```python
from build123d import *

# Parameters (mm, degrees)
BASE_FLANGE1_DEPTH = 490.75
CUT_EXTRUDE2_DEPTH = 514.204272196


# Sheet-metal steps are written as plain solids
with BuildPart() as part:
    # Sketch1 → Base-Flange1 (new, symmetric)
    with BuildSketch(Plane(origin=(0, 0, 0), x_dir=(1, 0, 0), z_dir=(0, 1, 0))):
        with BuildLine():
            Line((9.5, 58), (9.5, 68.0134))
            ThreePointArc((9.5, 68.0134), (10.081861668, 69.418138332), (11.4866, 70))
            Line((11.4866, 70), (37.5134, 70))
            ThreePointArc((37.5134, 70), (38.918138332, 69.418138332), (39.5, 68.0134))
            Line((39.5, 68.0134), (39.5, 23))
            Line((39.5, 23), (39.5, 18))
            Line((39.5, 18), (39.5, 7.8))
            ThreePointArc((39.5, 7.8), (41.269678139, 6.091041686), (42.915834526, 7.91928357))
            Line((42.915834526, 7.91928357), (42.359529101, 15.874821789))
            ThreePointArc((42.359529101, 15.874821789), (42.88838258, 17.368257942), (44.341289843, 18))
            Line((44.341289843, 18), (52.2634, 18))
            ThreePointArc((52.2634, 18), (53.668138332, 17.418138332), (54.25, 16.0134))
            Line((54.25, 16.0134), (54.25, -21.0134))
            ThreePointArc((54.25, -21.0134), (53.668138332, -22.418138332), (52.2634, -23))
            Line((52.2634, -23), (40.2366, -23))
            ThreePointArc((40.2366, -23), (39.715745145, -23.215745145), (39.5, -23.7366))
            Line((39.5, -23.7366), (39.5, -68.0134))
            ThreePointArc((39.5, -68.0134), (38.918138332, -69.418138332), (37.5134, -70))
            Line((37.5134, -70), (11.4866, -70))
            ThreePointArc((11.4866, -70), (10.081861668, -69.418138332), (9.5, -68.0134))
            Line((9.5, -68.0134), (9.5, -58))
            Line((9.5, -58), (10.75, -58))
            Line((10.75, -58), (10.75, -68.0134))
            ThreePointArc((10.75, -68.0134), (10.965745145, -68.534254855), (11.4866, -68.75))
            Line((11.4866, -68.75), (37.5134, -68.75))
            ThreePointArc((37.5134, -68.75), (38.034254855, -68.534254855), (38.25, -68.0134))
            Line((38.25, -68.0134), (38.25, -23.7366))
            ThreePointArc((38.25, -23.7366), (38.831861668, -22.331861668), (40.2366, -21.75))
            Line((40.2366, -21.75), (52.2634, -21.75))
            ThreePointArc((52.2634, -21.75), (52.784254855, -21.534254855), (53, -21.0134))
            Line((53, -21.0134), (53, 16.0134))
            ThreePointArc((53, 16.0134), (52.784254855, 16.534254855), (52.2634, 16.75))
            Line((52.2634, 16.75), (44.341289843, 16.75))
            ThreePointArc((44.341289843, 16.75), (43.802574707, 16.515759992), (43.606484164, 15.962017381))
            Line((43.606484164, 15.962017381), (44.162789589, 8.006479162))
            ThreePointArc((44.162789589, 8.006479162), (41.31330251, 4.841803152), (38.25, 7.8))
            Line((38.25, 7.8), (38.25, 18))
            Line((38.25, 18), (38.25, 23))
            Line((38.25, 23), (38.25, 68.0134))
            ThreePointArc((38.25, 68.0134), (38.034254855, 68.534254855), (37.5134, 68.75))
            Line((37.5134, 68.75), (11.4866, 68.75))
            ThreePointArc((11.4866, 68.75), (10.965745145, 68.534254855), (10.75, 68.0134))
            Line((10.75, 68.0134), (10.75, 58))
            Line((10.75, 58), (9.5, 58))
        make_face()
    extrude(amount=BASE_FLANGE1_DEPTH, both=True)

    # Sketch2 → Cut-Extrude2 (cut, through all)
    with BuildSketch(Plane.XY.offset(70)):
        Polygon((9.5, -490.75), (246.796446659, -253.453553341), (123.087268974, -490.75), align=None)
        Polygon((123.087268974, 490.75), (9.5, 490.75), (246.796446659, 253.453553341), align=None)
    extrude(amount=-CUT_EXTRUDE2_DEPTH, mode=Mode.SUBTRACT)


solid = part.part
```
Read the model definition and answer for the solid it produces. Units are mm, in the model's axes. A direction names the side the tool comes from. Coordinates: 2 decimals unless noted, no trailing zeros. Write each loop counter-clockwise with the first axis right and the second up, starting at its lowest first coordinate (ties: lowest second). Pieces come first, ordered by that corner, then holes. Notation, with made-up numbers: (-6, 13.5) - (12, 13.5) arc R21 ccw to (12, 49.5) - close; hole circle Ø10 at (51, -10). An arc over 180 degrees is marked (long way). Answer as a JSON object with one key per item and string values. Group by question number.
1. Which of the six approach directions +Z, -Z, +X, -X, +Y, -Y give full straight-line access (tool end or side, diameter ignored) to faces 1 (the flat face through (38.25, 6, 46)), 2 (the flat face through (39.5, 6, 46)), 3 (the flat face through (54.25, 6, 2))?
2. Consider L1, parallel to X at y = -132, z = -10; L2, parallel to Z at x = 22, y = 41; L3, parallel to X at y = 140, z = -6.5. Determine where each line is inside the solid, lowest interval first. Write a range as [from, to].
3. A cutting plane is placed at A-A (x = 24). Determine the outline of the cut face in (y, z), plus the area to 3 significant figures.
4. A cutting plane is placed at B-B (z = 39). Determine the outline of the cut face in (x, y), plus the area to 3 significant figures.
5. The mould has two halves that part along Z. Classify faces 4 (the flat face through (25, 7, -68.75)), 5 (the flat face through (25, 7, 70)), 6 (the flat face through (24, 7, -70)), 7 (the flat face through (43.37, -456.88, -10.04)): +Z half, -Z half, draft (parallel to the pull), parting line (faces both ways), or undercut.
6. Each of these flat-tipped pins is pushed along its axis until it touches: P1, Ø1.4, axis at x = 10, y = 37.5, coming from the +Z side; P2, Ø4, axis at x = 46.5, y = 36.5, coming from the +Z side; P3, Ø11, axis at y = 236, z = -63, coming from the +X side; P4, Ø1, axis at x = 40.5, z = 40.5, coming from the +Y side. Where does it stop, or does it pass through?
Worked out:
{
 "1": {"face 1": "+Y, -Y", "face 2": "+Z, +X, +Y, -Y", "face 3": "+Z, -Z, +X, +Y, -Y"},
 "2": {"L1": "x = [38.25, 39.5], [42.77, 44.02], [53, 54.25]", "L2": "z = [-70, -68.75], [68.75, 70]", "L3": "x = [38.55, 40.1], [42.32, 43.87], [53, 54.25]"},
 "3": {"outline": "(-476.25, -70) - (476.25, -70) - (476.25, -68.75) - (-476.25, -68.75) - close; (-476.25, 68.75) - (476.25, 68.75) - (476.25, 70) - (-476.25, 70) - close", "area": "2,380 mm²"},
 "4": {"outline": "(38.25, -462) - (39.5, -460.75) - (39.5, 460.75) - (38.25, 462) - close", "area": "1,150 mm²"},
 "5": {"face 4": "undercut", "face 5": "+Z half", "face 6": "-Z half", "face 7": "draft"},
 "6": {"P1": "stops at z = 69.84", "P2": "stops at z = 23", "P3": "stops at x = 39.5", "P4": "passes through"}
}
